Input: part model. Units: mm. Frame: model coordinates. Coordinates: 2 decimals unless noted, no trailing zeros. Order: outer loops, then holes, each group sorted by start corner. A loop starts at its lowest first (then second) coordinate and runs counter-clockwise, first axis right, second up. Notation, with made-up numbers: (38.25, 6.5) - (62.25, 6.5) arc R21 cw to (62.25, 25.5) - close; hole circle Ø11 at (-3.75, -9.75). An arc over 180 degrees is marked (long way). One line per question, with ' | ' between items.
from build123d import *

# Parameters (mm, degrees)
SKETCH1_R           = 8
SKETCH1_R_2         = 4.15
BOSS_EXTRUDE1_DEPTH = 5
CHAMFER1_SIZE       = 2.6
CHAMFER1_SIZE2      = 1.5011107
FILLET1_R           = 1


with BuildPart() as part:
    # Sketch1 → Boss-Extrude1 (new body)
    with BuildSketch(Plane(origin=(0, 0, 0), x_dir=(1, 0, 0), z_dir=(0, 1, 0))):
        Circle(SKETCH1_R)
        Circle(SKETCH1_R_2, mode=Mode.SUBTRACT)
    extrude(amount=BOSS_EXTRUDE1_DEPTH)

    # Chamfer1
    chamfer1_edges = [part.edges().sort_by_distance(p)[0] for p in [
        (-8, 5, 0),
    ]]
    chamfer1_side = [part.faces().sort_by_distance(p)[0] for p in [
        (-7.77372583, 5, 0),
    ]]
    chamfer(chamfer1_edges, length=CHAMFER1_SIZE, length2=CHAMFER1_SIZE2, reference=chamfer1_side[0])

    # Fillet1
    fillet1_edges = [part.edges().sort_by_distance(p)[0] for p in [
        (-8, 3.4988893, 0),
    ]]
    fillet(fillet1_edges, radius=FILLET1_R)


solid = part.part
Item 1: Draft query along Z for faces 1 (the face through (-0.9, 2.46, 4.05)), 2 (the face through (3.4, 0, 3.4)), 3 (the face through (5.11, 4.924, 2.119)). Return one class per face: released by +Z, released by -Z, zero draft, split by the parting line, or undercut.
Data:
face 1: undercut | face 2: zero draft | face 3: split by the parting line
Item 2: Section A-A on y = 1.15. Return the cut outline in (x, z).
Data:
outline: circle Ø16 at (0, 0); hole circle Ø8.3 at (0, 0)
Item 3: Ray query, line 1 (Z direction, x = 0, y = 1.2); line 2 (Z direction, x = 0, y = 3.3). Return the intervals inside material, ascending.
Data:
line 1: -8 to -4.15, 4.15 to 8 | line 2: -7.93 to -4.15, 4.15 to 7.93
